Check sheet for the modelled part. Datum: model origin and axes. Units: mm. A direction names the side the tool comes from. Give positions to 0.01 mm unless a question says otherwise; leave off trailing zeros. Order: outer loops, then holes, each group sorted by start corner. A loop starts at its lowest first (then second) coordinate and runs counter-clockwise, first axis right, second up. Notation, with made-up numbers: M 58.25,78 L 89.25,78 A22 cw 89.25,93 Z; hole C 89,21 d6. An arc over 180 degrees is marked long. Return JSON: item names as keys, results as strings. Group by question number.
from build123d import *

# Parameters (mm, degrees)
F0_W     = 10.5505171232
F0_H     = 5.8358493261
F1_DEPTH = 85
F3_DEPTH = 33.5
F4_D     = 4
F5_W     = 11.4551503211
F5_H     = 4.8642051406
F6_DEPTH = 42.7
F7_W     = 20
F7_H     = 50
F7_H_2   = 30
F8_DEPTH = 25


with BuildPart() as f1:
    # F0 (on Top) → F1 (new body)
    with BuildSketch(Plane.XY):
        with BuildLine():
            ThreePointArc((6.3000439482, -6.9552523798), (8.5786924555, -3.8042246479), (9.3843534363, 0))
            ThreePointArc((9.3843534363, 0), (8.5736712413, 3.8155275996), (6.2816887803, 6.9718344419))
            Line((6.2816887803, 6.9718344419), (-6.2816887803, 6.9718344419))
            ThreePointArc((-6.2816887803, 6.9718344419), (-9.384345286, 0.0123680735), (-6.3000439482, -6.9552523798))
            Line((-6.3000439482, -6.9552523798), (6.3000439482, -6.9552523798))
        make_face()
        with Locations((0.2029326279, 0)):
            Rectangle(F0_W, F0_H, mode=Mode.SUBTRACT)
        with BuildLine():
            ThreePointArc((6.2816887803, 6.9718344419), (8.5736712413, 3.8155275996), (9.3843534363, 0))
            ThreePointArc((9.3843534363, 0), (8.5786924555, -3.8042246479), (6.3000439482, -6.9552523798))
            Line((6.3000439482, -6.9552523798), (14.9059631667, -6.9552523798))
            Line((14.9059631667, -6.9552523798), (14.9059631667, 6.9718344419))
            Line((14.9059631667, 6.9718344419), (6.2816887803, 6.9718344419))
        make_face()
        with Locations((0.2029326279, 0)):
            Rectangle(F0_W, F0_H)
        with BuildLine():
            ThreePointArc((-6.3000439482, -6.9552523798), (-9.384345286, 0.0123680735), (-6.2816887803, 6.9718344419))
            Line((-6.2816887803, 6.9718344419), (-15.021123655, 6.9718344419))
            Line((-15.021123655, 6.9718344419), (-15.021123655, -6.9552523798))
            Line((-15.021123655, -6.9552523798), (-6.3000439482, -6.9552523798))
        make_face()
    extrude(amount=F1_DEPTH)

    # F3 (add): a face of the model
    f3_faces = [f1.faces().sort_by_distance(p)[0] for p in [
        (-0.0575802442, 0.008291031, 0),
    ]]
    extrude(f3_faces, amount=F3_DEPTH)

    # F4 (through all)
    with Locations(Plane.XZ.offset(6.9552523798)):
        with Locations((3.4722961341, 76.6178924305), (-3.4723085311, 76.6178924305), (3.4722961341, 59.8538924305), (-3.4723085311, 59.8538924305)):
            Hole(F4_D / 2)

    # F5 (on face) → F6 (join)
    with BuildSketch(Plane.XY.offset(85)):
        Rectangle(F5_W, F5_H)
    extrude(amount=F6_DEPTH)

    # F7 (on face) → F8 (cut)
    with BuildSketch(Plane.XZ.offset(6.9552523798)):
        with Locations((0, 25.75)):
            Rectangle(F7_W, F7_H)
        with Locations((0, -14.25)):
            Rectangle(F7_W, F7_H_2)
    extrude(amount=-F8_DEPTH, mode=Mode.SUBTRACT)


solid = f1.part
1) Release check for a two-part mould opening along Z. For faces 6 (the face through (0, 0, -33.5)), 7 (the face through (-10, 0, 11)), 8 (the face through (5.728, 0, 106)) record: released by +Z, released by -Z, zero draft, split by the parting line, or undercut.
2) Sectioned sample at A-A on x = 8.5. Record the boundary of the cut face in (y, z).
3) Depth check by flat-ended pin: P1, Ø1.5, axis at y = 0.5, z = 109, coming from the -X side; P2, Ø5.5, axis at y = 1, z = 104, coming from the +X side; P3, Ø12, axis at x = -9, z = 107, coming from the -Y side; P4, Ø3.5, axis at x = -3.47, z = 76.62, coming from the -Y side. Enter the tip coordinate at first touch or a pass-through.
4) Sectioned sample at C-C on x = -3.25. Record the boundary of the cut face in (y, z), then the cut area to 3 significant figures.
5) Sectioned sample at D-D on y = 1. Record the boundary of the cut face in (x, z), then the cut area to 3 significant figures.
6) Tool access check on faces 1 (the face through (10, 0, 10)), 2 (the face through (14.906, 0, 27)), 3 (the face through (0, 2.432, 106)), 4 (the face through (0, -2.432, 106)), 5 (the face through (-5.728, 0, 106)). Record the directions out of +Z, -Z, +X, -X, +Y, -Y that give a thin tool (end or side, any length) a straight path to the whole face; none if there is none.
7) Sectioned sample at B-B on z = -17.5. Record the boundary of the cut face in (x, y).
8) Material ranges on line 1 along Z through (x, y) = (3.75, 2.75); line 2 along Z through (x, y) = (3.5, 5.75); line 3 along X through (y, z) = (3.75, 9), recorded low to high.
Reply:
{
 "1": {"face 6": "released by -Z", "face 7": "undercut", "face 8": "zero draft"},
 "2": {"outline": "M -6.96,-33.5 L 6.97,-33.5 L 6.97,-29.25 L -6.96,-29.25 Z; M -6.96,50.75 L 6.97,50.75 L 6.97,85 L -6.96,85 Z"},
 "3": {"P1": "x = -5.73", "P2": "x = 5.73", "P3": "y = -2.43", "P4": "through"},
 "4": {"outline": "M -6.96,-33.5 L 6.97,-33.5 L 6.97,-29.25 L -6.96,-29.25 Z; M -6.96,50.75 L 6.97,50.75 L 6.97,57.87 L -6.96,57.87 Z; M -6.96,61.84 L 6.97,61.84 L 6.97,74.63 L -6.96,74.63 Z; M -6.96,78.61 L 6.97,78.61 L 6.97,85 L 2.43,85 L 2.43,127.7 L -2.43,127.7 L -2.43,85 L -6.96,85 Z", "area": "633 mm^2"},
 "5": {"outline": "M -15.02,-33.5 L 14.91,-33.5 L 14.91,85 L 5.73,85 L 5.73,127.7 L -5.73,127.7 L -5.73,85 L -15.02,85 Z; hole M -10,-29.25 L 10,-29.25 L 10,50.75 L -10,50.75 Z; hole C -3.47,59.85 d4; hole C -3.47,76.62 d4; hole C 3.47,59.85 d4; hole C 3.47,76.62 d4", "area": "2,390 mm^2"},
 "6": {"face 1": "+Y, -Y", "face 2": "+Z, -Z, +X, +Y, -Y", "face 3": "+Z, +X, -X, +Y", "face 4": "+Z, +X, -X, -Y", "face 5": "+Z, -X, +Y, -Y"},
 "7": {"outline": "M -15.02,-6.96 L -10,-6.96 L -10,6.97 L -15.02,6.97 Z; M 10,-6.96 L 14.91,-6.96 L 14.91,6.97 L 10,6.97 Z"},
 "8": {"line 1": "-33.5 to -29.25, 50.75 to 57.87, 61.83 to 74.64, 78.6 to 85", "line 2": "-33.5 to -29.25, 50.75 to 57.85, 61.85 to 74.62, 78.62 to 85", "line 3": "-15.02 to -10, 10 to 14.91"}
}
